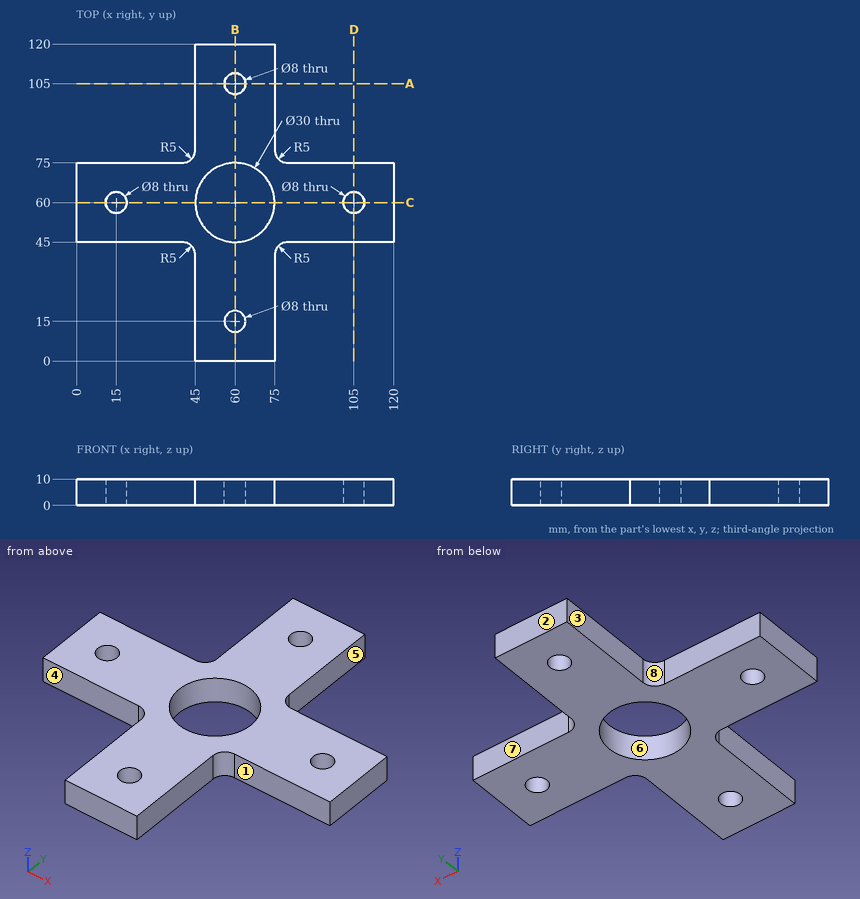
Can you work these out from the drawing? Everything is in mm from the part's minimum corner. A direction names the side the tool comes from. Coordinates: 2 decimals unless noted, no trailing zeros. Write each loop counter-clockwise with the first axis right and the second up, starting at its lowest first coordinate (ties: lowest second). Pieces come first, ordered by that corner, then holes. Notation, with made-up numbers: (-1, 31.5) -> (18, 31.5) arc R19 ccw to (18, 67.5) -> close; hole circle Ø2 at (-6.5, 75). An arc over 180 degrees is marked (long way). Write each question's results on one line, items separated by ' | '. Start each with the question number.
Q1. I'm going to push flat-ended pins straight in: pin 1 (2 mm diameter, centred on y = 13, z = 6.5, fed in from +X); pin 2 (5 mm diameter, centred on x = 109, z = 5.5, fed in from +Y); pin 3 (7 mm diameter, centred on x = 60, y = 105, fed in from -Z); pin 4 (5 mm diameter, centred on y = 95.5, z = 7, fed in from -X). Where does each tip first touch, or does it pass through?
Q2. If I drill on probe 1 along Y at (x, z) = (60.5, 9.5); probe 2 along Y at (x, z) = (61, 6.5); probe 3 along Y at (x, z) = (105, 2.5), over which ranges is the centre line in solid material (lowest first)?
Q3. Imagine slicing it at A-A (y = 105). Write out the boundary of the cut face in (x, z).
Q4. We'd pull the mould along X, two halves only. Please class the marked faces 6, 7 and 8: +X half, -X half, draft (parallel to the pull), parting line (faces both ways), or undercut.
Q5. Imagine slicing it at B-B (x = 60). Write out the boundary of the cut face in (y, z).
Q6. On a 3-axis mill with a long thin cutter (end or side, diameter ignored), from which of +Z, -Z, +X, -X, +Y, -Y can I reach the whole of each face in a straight line? I mean the marked faces 1, 2, 3, 4 and 5. Say none if no direction works.
Taken from the geometry:
1) pin 1: stops at x = 75 | pin 2: stops at y = 75 | pin 3: passes through | pin 4: stops at x = 45
2) probe 1: y = 0 to 11.03, 18.97 to 45.01, 74.99 to 101.03, 108.97 to 120 | probe 2: y = 0 to 11.13, 18.87 to 45.03, 74.97 to 101.13, 108.87 to 120 | probe 3: y = 45 to 56, 64 to 75
3) outline: (45, 0) -> (56, 0) -> (56, 10) -> (45, 10) -> close; (64, 0) -> (75, 0) -> (75, 10) -> (64, 10) -> close
4) face 6: undercut | face 7: draft | face 8: -X half
5) outline: (0, 0) -> (11, 0) -> (11, 10) -> (0, 10) -> close; (19, 0) -> (45, 0) -> (45, 10) -> (19, 10) -> close; (75, 0) -> (101, 0) -> (101, 10) -> (75, 10) -> close; (109, 0) -> (120, 0) -> (120, 10) -> (109, 10) -> close
6) face 1: +Z, -Z, +X, -Y | face 2: +Z, -Z, +X, -X, +Y | face 3: +Z, -Z, -X, +Y | face 4: +Z, -Z, -X, -Y | face 5: +Z, -Z, +X, +Y
